Verification items for the finished model (mm, model axes). A direction names the side the tool comes from. Round coordinates to 2 decimals unless told otherwise and drop trailing zeros. Write each loop counter-clockwise with the first axis right and the second up, starting at its lowest first coordinate (ties: lowest second). Pieces come first, ordered by that corner, then holes. Notation, with made-up numbers: (8, 51) - (58, 51) arc R29 cw to (58, 90) - close; hole circle Ø5 at (18, -3.5). An arc over 180 degrees is marked (long way). Answer as a JSON object with one key per item and string values.
```python
from build123d import *

# Parameters (mm, degrees)
SKETCH_1_W          = 30
SKETCH_1_H          = 30
EXTRUDE_1_DEPTH     = 50
SKETCH_3_W          = 30
SKETCH_3_H          = 87.301509621
EXTRUDE_2_DEPTH     = 40
SKETCH_4_W          = 30
SKETCH_4_H          = 77.301509621
EXTRUDE_3_DEPTH     = 30
SKETCH_7_W          = 40
SKETCH_7_H          = 10
CUT_EXTRUDE_1_DEPTH = 30
CUT_EXTRUDE_2_DEPTH = 30
CUT_EXTRUDE_5_DEPTH = 30
SKETCH_21_R         = 3
CUT_EXTRUDE_6_DEPTH = 50


with BuildPart() as part:
    # 草图1 → 凸台-拉伸1 (new body)
    with BuildSketch(Plane(origin=(0, 0, 0), x_dir=(1, 0, 0), z_dir=(0, 1, 0))):
        Rectangle(SKETCH_1_W, SKETCH_1_H)
    extrude(amount=EXTRUDE_1_DEPTH)

    # 草图3 → 凸台-拉伸2 (add)
    with BuildSketch(Plane.ZY.offset(15)):
        with Locations((0, -33.650754811)):
            Rectangle(SKETCH_3_W, SKETCH_3_H)
    extrude(amount=EXTRUDE_2_DEPTH)

    # 草图4 → 凸台-拉伸3 (add)
    with BuildSketch(Plane(origin=(-15, 0, 0), x_dir=(0, 0, -1), z_dir=(1, 0, 0))):
        with Locations((0, -38.650754811)):
            Rectangle(SKETCH_4_W, SKETCH_4_H)
    extrude(amount=EXTRUDE_3_DEPTH)

    # 草图7 → 切除-拉伸1 (cut)
    with BuildSketch(Plane.XY.offset(15)):
        with Locations((-35, 5)):
            Rectangle(SKETCH_7_W, SKETCH_7_H)
    extrude(amount=-CUT_EXTRUDE_1_DEPTH, mode=Mode.SUBTRACT)

    # 草图8 → 切除-拉伸2 (cut)
    with BuildSketch(Plane.XY.offset(15)):
        Polygon((-15, 0), (-55, 0), (-95.241358959, -77.747534748), (-55.241358959, -77.747534748), align=None)
    extrude(amount=-CUT_EXTRUDE_2_DEPTH, mode=Mode.SUBTRACT)

    # 草图9 → 切除-拉伸5 (cut)
    with BuildSketch(Plane.XY.offset(15)):
        Polygon((15, 0), (-26.125228954, -79.582689845), (25.626144769, -79.582689845), (66.751373723, 0), align=None)
    extrude(amount=-CUT_EXTRUDE_5_DEPTH, mode=Mode.SUBTRACT)

    # 草图21 → 切除-拉伸6 (cut)
    with BuildSketch(Plane(origin=(0, 50, 0), x_dir=(1, 0, 0), z_dir=(0, 1, 0))):
        with Locations(Location((0, 0, 0), (0, 0, 270))):
            Circle(SKETCH_21_R)
    extrude(amount=-CUT_EXTRUDE_6_DEPTH, mode=Mode.SUBTRACT)


solid = part.part
```
Q1. Material ranges on line 1 along X through (y, z) = (38, 0); line 2 along X through (y, z) = (11.5, 0.75); line 3 along X through (y, z) = (10.5, -4.25), recorded low to high. Write a range as [from, to].
Geometry check:
{"line 1": "x = [-15, -3], [3, 15]", "line 2": "x = [-15, -2.9], [2.9, 15]", "line 3": "x = [-15, 15]"}
Q2. Set-up check for faces 1 (the flat face through (-15, 25, 0)), 2 (the flat face through (-40, -77.302, 0)): record each of +Z, -Z, +X, -X, +Y, -Y from which the full face is reachable in a straight line by a thin tool's end or side.
Geometry check:
{"face 1": "+Z, -Z, -X, +Y", "face 2": "+Z, -Z, +X, -X, -Y"}
Q3. Section check D-D, the plane y = -35.5. Record the cut outline in (x, z).
Geometry check:
{"outline": "(-33.37, -15) - (-3.35, -15) - (-3.35, 15) - (-33.37, 15) - close"}
Q4. Section check C-C, the plane x = 0. Record the cut outline in (y, z), then the cut area to 3 significant figures.
Geometry check:
{"outline": "(-29.03, -15) - (50, -15) - (50, -3) - (0, -3) - (0, 3) - (50, 3) - (50, 15) - (-29.03, 15) - close", "area": "2,070 mm2"}
Q5. Section check B-B, the plane y = 17. Record the cut outline in (x, z), then the cut area to 3 significant figures.
Geometry check:
{"outline": "(-15, -15) - (15, -15) - (15, 15) - (-15, 15) - close; hole circle Ø6 at (0, 0)", "area": "872 mm2"}
Q6. Gauge pin test, flat ends, axial feed: P1, Ø1.5, axis at y = -28.5, z = 6.5, coming from the +X side; P2, Ø1, axis at y = -11, z = 5.5, coming from the -X side; P3, Ø9.5, axis at x = 0, z = 0, coming from the -Y side. Record the tip position at first contact, or that the pin passes through.
Geometry check:
{"P1": "stops at x = 0.66", "P2": "stops at x = -20.95", "P3": "stops at y = -38.22"}
Q7. Release check for a two-part mould opening along X. For faces 3 (the flat face through (0, 0, 0)), 4 (the flat face through (-4, 50, 0)), 5 (the cylindrical face through (0.9, 25.35, 2.86)), 6 (the flat face through (-4.694, -38.11, 0.21)) record: released by +X, released by -X, zero draft, split by the parting line, or undercut.
Geometry check:
{"face 3": "undercut", "face 4": "zero draft", "face 5": "undercut", "face 6": "released by +X"}
